Autodesk Inventor part; units mm, degrees
ref_plane "YZ Plane" through (0, 0, 0) normal (1, 0, 0) x (0, 1, 0)
ref_plane "XZ Plane" through (0, 0, 0) normal (0, 1, 0) x (-1, 0, 0)
ref_plane "XY Plane" through (0, 0, 0) normal (0, 0, 1) x (1, 0, 0)
sketch "Sketch1" plane through (0, 0, 0) normal (0, 1, 0) x (-1, 0, 0)
  line L0 (-2.0311, -3.494) -> (-4.0414, 0.012)
  line L1 (-4.0414, 0.012) -> (-2.0104, 3.506)
  line L2 (-2.0104, 3.506) -> (2.0311, 3.494)
  line L3 (2.0311, 3.494) -> (4.0414, -0.012)
  line L4 (4.0414, -0.012) -> (2.0104, -3.506)
  line L5 (2.0104, -3.506) -> (-2.0311, -3.494)
  point P0 (0, 0)
  point P1 (0, 0)
  dimension "d0" = 7
extrude "Extrusion1" add sketch "Sketch1" along normal blind 2
sketch "Sketch2" plane through (0, 2, 0) normal (0, 1, 0) x (1, 0, 0)
  circle A0 centre (0, 0) radius 2.5
  dimension "d3" = 5
extrude "Extrusion2" add sketch "Sketch2" along normal blind 15
sketch "Sketch3" plane through (0, 17, 0) normal (0, 1, 0) x (1, 0, 0)
  point P0 (0, 0)
properties part number "Screw 5 mm"
CAD build for the part. Positions are in the model's coordinates, mm. A direction names the side the tool comes from. Coordinates: 2 decimals unless noted, no trailing zeros. Order: outer loops, then holes, each group sorted by start corner. A loop starts at its lowest first (then second) coordinate and runs counter-clockwise, first axis right, second up. Notation, with made-up numbers: (-35, 69.25) - (-7, 69.25) arc R19 ccw to (-7, 93.25) - close; hole circle Ø2 at (37, 89.5). An arc over 180 degrees is marked (long way). Use a Markdown table: item, result. Add a question column.
(1) Flat gauge pins, fed straight in: pin 1 (1 mm diameter, centred on x = -0.5, z = 0.5, fed in from -Y); pin 2 (2 mm diameter, centred on y = 9, z = -1, fed in from +X); pin 3 (4 mm diameter, centred on y = 13.5, z = 1.5, fed in from -X); pin 4 (3 mm diameter, centred on x = -3, y = 4.5, fed in from -Z). Where does each tip first touch, or does it go through?
(2) Saw through at D-D (z = -2.75). Give the cut face in (x, y), then the cut area to 3 significant figures.
(3) Which spindle directions (+Z, -Z, +X, -X, +Y, -Y) get a long thin tool onto all of the face, cutting with end or side? Do faces 1 (the face through (0, 0, 0)), 2 (the face through (-0.54, 9.4, -2.44)). Say none if no direction does.
(4) Saw through at C-C (y = 7.75). Give the cut face in (x, z), then the cut area to 3 significant figures.
(5) Drill centre lines: line 1 along Y through (x, z) = (-3, -0.75); line 2 along X through (y, z) = (7.75, 0); line 3 along Z through (x, y) = (-0.5, 16). Where is each one in solid material? Low to high. Write a range as [from, to].
(6) Saw through at A-A (z = -0.5). Give the cut face in (x, y).
(7) Saw through at B-B (x = -1.5). Give the cut face in (y, z).
Solved:
| question | item | result |
|---|---|---|
| 1 | pin 1 | stops at y = 0 |
| 1 | pin 2 | stops at x = 2.5 |
| 1 | pin 3 | stops at x = -2.5 |
| 1 | pin 4 | stops at z = -2 |
| 2 | outline | (-2.45, 0) - (2.46, 0) - (2.46, 2) - (-2.45, 2) - close |
| 2 | area | 9.82 mm² |
| 3 | face 1 | +Z, -Z, +X, -X, -Y |
| 3 | face 2 | +Y |
| 4 | outline | circle Ø5 at (0, 0) |
| 4 | area | 19.6 mm² |
| 5 | line 1 | y = [0, 2] |
| 5 | line 2 | x = [-2.5, 2.5] |
| 5 | line 3 | z = [-2.45, 2.45] |
| 6 | outline | (-3.76, 0) - (3.75, 0) - (3.75, 2) - (2.45, 2) - (2.45, 17) - (-2.45, 17) - (-2.45, 2) - (-3.76, 2) - close |
| 7 | outline | (0, -3.5) - (2, -3.5) - (2, -2) - (17, -2) - (17, 2) - (2, 2) - (2, 3.5) - (0, 3.5) - close |
